The model under review builds one solid part; all positions refer to its coordinate system, in mm. Face numbers are marked on the shaded views. A direction names the side the tool comes from. Coordinates: 2 decimals unless noted, no trailing zeros. Order: outer loops, then holes, each group sorted by start corner. A loop starts at its lowest first (then second) coordinate and runs counter-clockwise, first axis right, second up. Notation, with made-up numbers: M 58,59.25 L 108,59.25 A36 cw 108,98.25 Z; hole C 86.25,-11 d6. An arc over 180 degrees is marked long. Answer as CSV lines item,"result". Start each with the question number.
Q1. Consider section A-A on x = -9.5. Write out the cut boundary in (y, z), and give its area (3 significant figures).
Q2. Machinability: for the marked faces 1, 2, 3 and 4, which of the approach directions +Z, -Z, +X, -X, +Y, -Y give a long, thin tool a straight path to every point of the face, cutting with its end or side? Answer none if there is none.
Q3. Consider section B-B on y = 8. Write out the cut boundary in (x, z), and give its area (3 significant figures).
Q4. For P1, Ø3, axis at y = -21, z = 40.5, coming from the +X side; P2, Ø15, axis at x = 1, y = 4.5, coming from the +Z side; P3, Ø1.6, axis at y = -26, z = 40.5, coming from the +X side, all flat-tipped, find the tip position at first contact; note any pin that passes through.
Q5. The part is to be moulded in two halves that separate along X. For the marked faces 5, 6, 7 and 8, say which applies: +X half, -X half, draft (parallel to the pull), parting line (faces both ways), or undercut.
Q6. Consider section C-C on x = 23.5. Write out the cut boundary in (y, z), and give its area (3 significant figures).
Q7. Consider section D-D on y = -23.91. Write out the cut boundary in (x, z), and give its area (3 significant figures).
Q8. Wall thickness on L1, parallel to X at y = 27.5, z = 23; L2, parallel to Y at x = -9, z = 26.5; L3, parallel to X at y = 11, z = 15.5: over which ranges is each line inside the solid? List them lowest first. Write a range as [from, to].
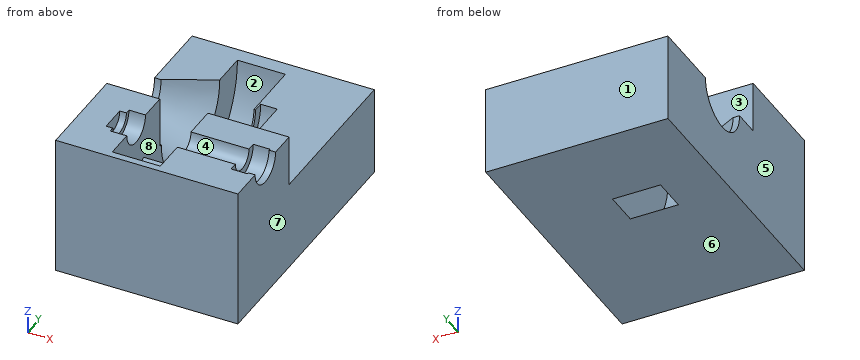
Solid Edge part; units mm, degrees
sketch "Sketch1" plane through (0, 0, 0) normal (0, 0, 1) x (1, 0, 0)
  line L0 (-28, -40) -> (28, -40)
  line L1 (28, -40) -> (28, 40)
  line L2 (28, 40) -> (-28, 40)
  line L3 (-28, 40) -> (-28, -40)
  dimension "D1" = 28
  dimension "D2" = 28
extrude "Protrusion1" add sketch "Sketch1" along normal blind 60
sketch "Sketch2" plane through (28, 0, 30) normal (1, 0, 0) x (0, 1, 0)
  line L0 (-10, 30) -> (-10, -3)
  line L1 (-10, -3) -> (40, -3)
  dimension "D1" = 10
extrude "Extrusionsausschnitt_1" cut sketch "Sketch2" against normal blind 62 material side at (28, -9.95, 43.5)
sketch "Sketch3" plane through (28, 0, 30) normal (1, 0, 0) x (0, 1, 0)
  line L0 (-40, 12.56) -> (-10, 12.56)
extrude "Extrusionsausschnitt_2" cut sketch "Sketch3" against normal blind 92 material side at (28, -25, 42.61)
sketch "Sketch4" plane through (8, 0, 21.28) normal (-1, 0, 0) x (0, -1, 0)
  circle A0 centre (-8, 5.72) radius 12
extrude "Extrusionsausschnitt_3" cut sketch "Sketch4" along normal blind 5
sketch "Sketch5" plane through (3, 5.5, 20.5) normal (1, 0, 0) x (0, 1, 0)
  circle A0 centre (2.5, 6.5) radius 9
extrude "Extrusionsausschnitt_4" cut sketch "Sketch5" against normal blind 1.5
sketch "Sketch6" plane through (1.5, 5.5, 22.5) normal (1, 0, 0) x (0, 1, 0)
  circle A0 centre (2.5, 4.5) radius 27.5
extrude "Extrusionsausschnitt_5" cut sketch "Sketch6" against normal blind 13.5
sketch "Sketch7" plane through (1.5, 5.5, 21.28) normal (-1, 0, 0) x (0, 0, 1)
  circle A0 centre (5.72, 2.5) radius 27.5
extrude "Extrusionsausschnitt_6" cut sketch "Sketch7" against normal blind 1
sketch "Sketch8" plane through (0, 15, 27) normal (0, 0, 1) x (1, 0, 0)
  line L0 (-12, 10.1524) -> (-28, 2)
  line L1 (-12, 10.1524) -> (-12, -7)
revolve "RevolvedCutout1" cut sketch "Sketch8" angle 360 about axis through (-28, 8, 27) along (1, 0, 0) material side at (-19.9773, 21.0316, 27)
sketch "Sketch9" plane through (-28, 0, 21.28) normal (-1, 0, 0) x (0, -1, 0)
  circle A0 centre (-8, 5.72) radius 10
extrude "Cutout1" cut sketch "Sketch9" against normal up to vertex (16 mm away)
sketch "Sketch10" plane through (-12, 0, 21.28) normal (-1, 0, 0) x (0, 0, 1)
  circle A0 centre (21.28, -23.91) radius 14
extrude "Extrusionsausschnitt_8" cut sketch "Sketch10" against normal up to vertex (14.5 mm away)
sketch "Sketch11" plane through (-12, -0.75, 21.28) normal (1, 0, 0) x (0, 1, 0)
  circle A0 centre (-23.16, 21.28) radius 5.5
extrude "Extrusionsausschnitt_9" cut sketch "Sketch11" against normal blind 5
sketch "Sketch12" plane through (-17, -23.91, 39.81) normal (1, 0, 0) x (0, 1, 0)
  circle A0 centre (0, 2.75) radius 4
extrude "Extrusionsausschnitt_10" cut sketch "Sketch12" against normal blind 2
sketch "Sketch13" plane through (2.5, -0.75, 21.28) normal (-1, 0, 0) x (0, -1, 0)
  circle A0 centre (23.16, 21.28) radius 4
extrude "Extrusionsausschnitt_11" cut sketch "Sketch13" against normal blind 17.5
sketch "Sketch14" plane through (20, -23.91, 40.56) normal (-1, 0, 0) x (0, -1, 0)
  circle A0 centre (0, 2) radius 6.5
extrude "Extrusionsausschnitt_12" cut sketch "Sketch14" against normal blind 5
sketch "Sketch15" plane through (25, -23.91, 38.81) normal (-1, 0, 0) x (0, -1, 0)
  circle A0 centre (0, 3.75) radius 6
extrude "Extrusionsausschnitt_13" cut sketch "Sketch15" against normal blind 24
sketch "Sketch16" plane through (28, 0, 21.28) normal (1, 0, 0) x (0, 1, 0)
  circle A0 centre (-23.6974, 21.295) radius 9.5
extrude "Extrusionsausschnitt_14" cut sketch "Sketch16" against normal blind 1
sketch "Sketch17" plane through (15.25, -14.955, 42.56) normal (0, 0, 1) x (1, 0, 0)
  line L0 (11.75, 54.955) -> (11.75, -25.045)
extrude "Extrusionsausschnitt_15" cut sketch "Sketch17" against normal blind 100 material side at (27.05, 0, 42.56)
properties material "Aluminiumlegierung:3.0205, Al 99.0, EN-AW 1200"
Evaluation:
1,outline,"M -40,0 L 2.78,0 A27.5 cw -19.4,29.31 A14 cw -37.91,42.56 L -40,42.56 Z; M 13.22,0 L 40,0 L 40,27 L 35.5,27 A27.5 cw Z"
1,area,"1,080 mm²"
2,face 1,"+Z, -Z, +X, -X, +Y"
2,face 2,"+Z"
2,face 3,"+Z, +X, -X, +Y"
2,face 4,"+Z, +X"
3,outline,"M -28,0 L -12,0 L -12,9.85 L -26.04,17 L -28,17 Z; M 2.5,0 L 27,0 L 27,27 L 8,27 L 8,15 L 3,15 L 3,18 L 2.5,18 Z"
3,area,"819 mm²"
4,P1,"stops at x = 20"
4,P2,"stops at z = 27"
4,P3,"stops at x = -19"
5,face 5,"-X half"
5,face 6,"draft"
5,face 7,"+X half"
5,face 8,"undercut"
6,outline,"M -40,0 L 40,0 L 40,27 L -10,27 L -10,42.56 L -17.41,42.56 A6.5 cw -30.41,42.56 L -40,42.56 Z"
6,area,"2,560 mm²"
7,outline,"M -28,0 L 27,0 L 27,36.56 L 25,36.56 L 25,36.06 L 20,36.06 L 20,38.56 L 2.5,38.56 L 2.5,28.56 L -12,28.56 L -12,37.06 L -17,37.06 L -17,38.56 L -19,38.56 L -19,42.56 L -28,42.56 Z"
7,area,"1,990 mm²"
8,L1,"x = [-28, -12], [2.5, 27]"
8,L2,"y = [-40, -19.5], [35.5, 40]"
8,L3,"x = [-28, -22.34], [2.5, 3], [8, 27]"
